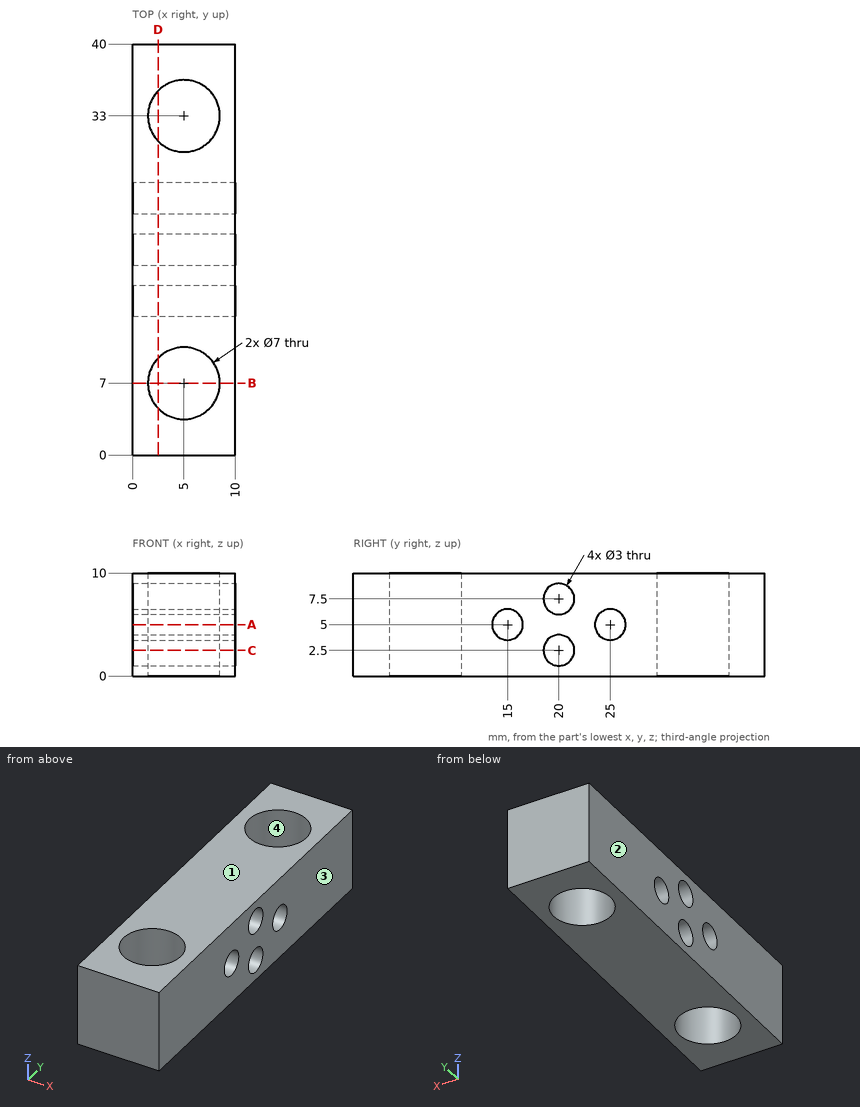
For this review, use the dimensioned drawing (mm, ordinates from the lowest corner) and the shaded views. Round coordinates to 2 decimals unless told otherwise and drop trailing zeros. Write each loop counter-clockwise with the first axis right and the second up, starting at its lowest first coordinate (ties: lowest second). Pieces come first, ordered by that corner, then holes. Notation, with made-up numbers: M -32.5,51.25 L -25.5,51.25 A21 cw -25.5,78.25 Z; hole C -12.5,66.25 d10. An arc over 180 degrees is marked long. Answer as CSV lines item,"result". Start each with the question number.
Q1. Consider section C-C, the plane z = 2.5. Give the boundary of the cut face in (x, y).
Q2. Consider section B-B, the plane y = 7. Give the boundary of the cut face in (x, z), then the cut area to 3 significant figures.
Q3. Wall thickness on line 1 along Z through (x, y) = (1.5, 15); line 2 along Z through (x, y) = (9, 19.5); line 3 along Y through (x, z) = (5.25, 3.75): over which ranges is each line inside the solid? List them lowest first.
Q4. The part is to be moulded in two halves that separate along X. For the marked faces 1, 2, 3 and 4, say which applies: +X half, -X half, draft (parallel to the pull), parting line (faces both ways), or undercut.
Q5. Consider section D-D, the plane x = 2.5. Give the boundary of the cut face in (y, z), then the cut area to 3 significant figures.
Q6. Consider section A-A, the plane z = 5. Give the boundary of the cut face in (x, y), then the cut area to 3 significant figures.
Result set:
1,outline,"M 0,0 L 10,0 L 10,18.5 L 0,18.5 Z; M 0,21.5 L 10,21.5 L 10,40 L 0,40 Z; hole C 5,7 d7; hole C 5,33 d7"
2,outline,"M 0,0 L 1.5,0 L 1.5,10 L 0,10 Z; M 8.5,0 L 10,0 L 10,10 L 8.5,10 Z"
2,area,"30.0 mm²"
3,line 1,"z = 0 to 3.5, 6.5 to 10"
3,line 2,"z = 0 to 1.09, 3.91 to 6.09, 8.91 to 10"
3,line 3,"y = 0 to 3.51, 10.49 to 14.17, 15.83 to 19.17, 20.83 to 24.17, 25.83 to 29.51, 36.49 to 40"
4,face 1,"draft"
4,face 2,"-X half"
4,face 3,"+X half"
4,face 4,"undercut"
5,outline,"M 0,0 L 4.55,0 L 4.55,10 L 0,10 Z; M 9.45,0 L 30.55,0 L 30.55,10 L 9.45,10 Z; M 35.45,0 L 40,0 L 40,10 L 35.45,10 Z; hole C 15,5 d3; hole C 20,2.5 d3; hole C 20,7.5 d3; hole C 25,5 d3"
5,area,"274 mm²"
6,outline,"M 0,0 L 10,0 L 10,13.5 L 0,13.5 Z; M 0,16.5 L 10,16.5 L 10,23.5 L 0,23.5 Z; M 0,26.5 L 10,26.5 L 10,40 L 0,40 Z; hole C 5,7 d7; hole C 5,33 d7"
6,area,"263 mm²"
